Design review of the part shown in the three views and the two pictorial views. Dimensions are in mm from the part's minimum x, y and z. A direction names the side the tool comes from. Round coordinates to 2 decimals unless told otherwise and drop trailing zeros. Loops run counter-clockwise (first coordinate to the right, second up) from the corner with the lowest first, then second, coordinate; pieces in that order, holes last. Notation, with made-up numbers: (44, 38) - (89, 38) arc R18 ccw to (89, 58) - close; hole circle Ø11 at (-6.75, 45). An arc over 180 degrees is marked (long way). Return JSON: item names as keys, results as strings. Group by question number.
(1) We need section B-B, the plane z = 45. Write out the cut boundary in (x, y), and give its area (3 significant figures).
(2) The part is to be moulded in two halves that separate along X. For the marked faces 3, 4 and 5, say which applies: pulls with the +X half, pulls with the -X half, needs draft (parallel to the pull), parting line crosses it, or undercut.
(3) We need section D-D, the plane y = 31. Write out the cut boundary in (x, z).
(4) We need section A-A, the plane y = 43. Write out the cut boundary in (x, z), and give its area (3 significant figures).
(5) Clearance check with flat-ended pins moving along their axes: pin 1 (4.5 mm diameter, centred on y = 7, z = 45, fed in from -X); pin 2 (1 mm diameter, centred on x = 71, y = 37.5, fed in from +Z); pin 3 (8 mm diameter, centred on y = 7, z = 45, fed in from +X). State where each tip first meets the part, or that it passes through.
(6) We need section C-C, the plane z = 32. Write out the cut boundary in (x, y), and give its area (3 significant figures).
(7) Wall thickness on L1, parallel to Y at x = 93.4, z = 45; L2, parallel to Z at x = 92.3, y = 7; L3, parallel to X at y = 21.5, z = 33: over which ranges is each line inside the solid? List them lowest first. Write a range as [from, to].
(8) For the marked faces 1 and 2, list the 3-axis set-ups (+Z, -Z, +X, -X, +Y, -Y) from which the entire face can be reached by the end or side of a thin tool; tool diameter is ignored.
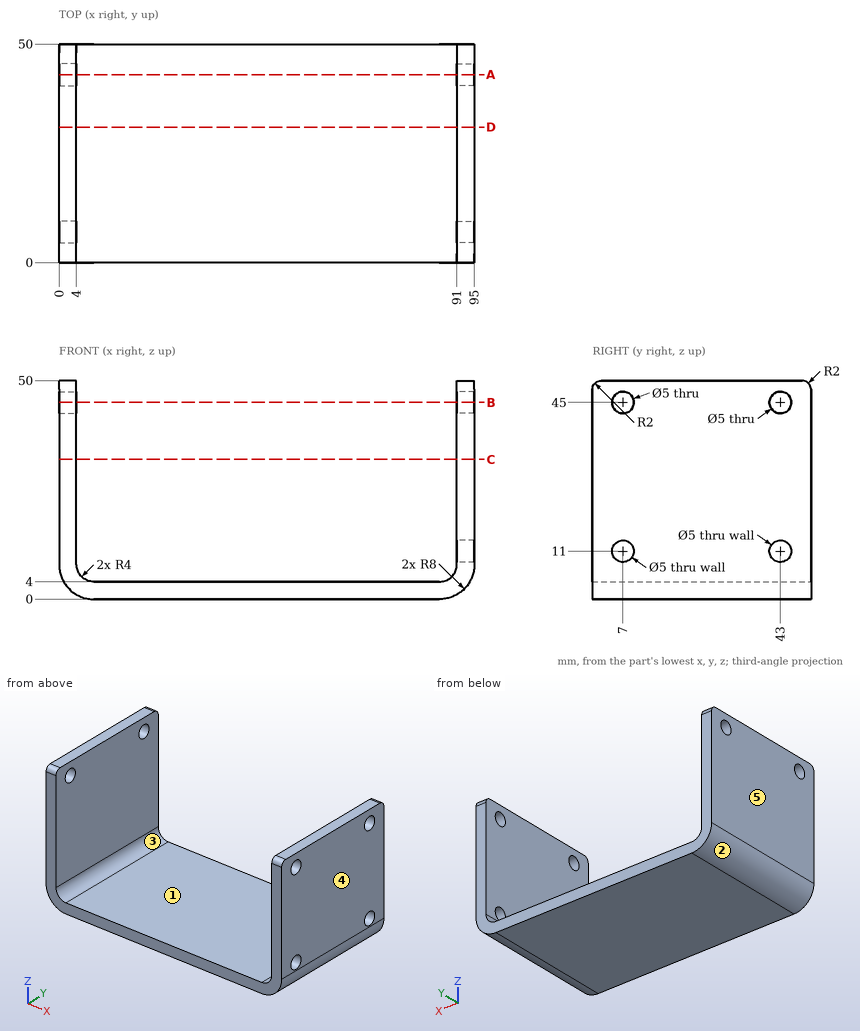
Solutions:
{
 "1": {"outline": "(0, 0) - (4, 0) - (4, 4.5) - (0, 4.5) - close; (0, 9.5) - (4, 9.5) - (4, 40.5) - (0, 40.5) - close; (0, 45.5) - (4, 45.5) - (4, 50) - (0, 50) - close; (91, 0) - (95, 0) - (95, 4.5) - (91, 4.5) - close; (91, 9.5) - (95, 9.5) - (95, 40.5) - (91, 40.5) - close; (91, 45.5) - (95, 45.5) - (95, 50) - (91, 50) - close", "area": "320 mm^2"},
 "2": {"face 3": "undercut", "face 4": "pulls with the +X half", "face 5": "pulls with the -X half"},
 "3": {"outline": "(0, 8) arc R8 ccw to (8, 0) - (87, 0) arc R8 ccw to (95, 8) - (95, 50) - (91, 50) - (91, 8) arc R4 cw to (87, 4) - (8, 4) arc R4 cw to (4, 8) - (4, 50) - (0, 50) - close"},
 "4": {"outline": "(0, 8) arc R8 ccw to (8, 0) - (87, 0) arc R8 ccw to (95, 8) - (95, 8.5) - (91, 8.5) - (91, 8) arc R4 cw to (87, 4) - (8, 4) arc R4 cw to (4, 8) - (4, 42.5) - (0, 42.5) - close; (0, 47.5) - (4, 47.5) - (4, 50) - (0, 50) - close; (91, 13.5) - (95, 13.5) - (95, 42.5) - (91, 42.5) - close; (91, 47.5) - (95, 47.5) - (95, 50) - (91, 50) - close", "area": "667 mm^2"},
 "5": {"pin 1": "through", "pin 2": "z = 4", "pin 3": "x = 95"},
 "6": {"outline": "(0, 0) - (4, 0) - (4, 50) - (0, 50) - close; (91, 0) - (95, 0) - (95, 50) - (91, 50) - close", "area": "400 mm^2"},
 "7": {"L1": "[0, 4.5], [9.5, 40.5], [45.5, 50]", "L2": "[2.01, 8.5], [13.5, 42.5], [47.5, 50]", "L3": "[0, 4], [91, 95]"},
 "8": {"face 1": "+Z, +Y, -Y", "face 2": "-Z, -X, +Y, -Y"}
}
